Work out the finished part from the listing and answer in its coordinate system (mm). Coordinates: 2 decimals unless noted, no trailing zeros. Write each loop counter-clockwise with the first axis right and the second up, starting at its lowest first coordinate (ties: lowest second). Pieces come first, ordered by that corner, then holes. Notation, with made-up numbers: (1.5, -39) - (42.5, -39) arc R18 cw to (42.5, -26) - close; hole circle Ø6 at (78.5, 80.25). An arc over 180 degrees is marked (long way). Use a Markdown table: item, result. Add a question column.
(1) The part is cut by section C-C, the plane z = 1.55. Give the vertices of the cut face in (x, y), then the cut area to 3 significant figures.
(2) The part is cut by section A-A, the plane y = 0. Give the vertices of the cut face in (x, z), then the cut area to 3 significant figures.
(3) Find the intervals of material crossed by line 1 (Y direction, x = 0, z = 0.8); line 2 (Y direction, x = -30, z = 1.05); line 3 (X direction, y = -8, z = 2.4), in increasing order. Write a range as from..to.
(4) Given pin 1 Ø1.5 at (y, z) = (-8.5, 2) entering from -X; pin 2 Ø0.8 at (y, z) = (13.5, 1.5) entering from -X; pin 3 Ø1.2 at (y, z) = (11, 1) entering from +X, each flat-ended and moving along its own axis, determine where each tip first touches the part or whether it passes through.
(5) The part is cut by section D-D, the plane x = 9.5. Give the vertices of the cut face in (y, z).
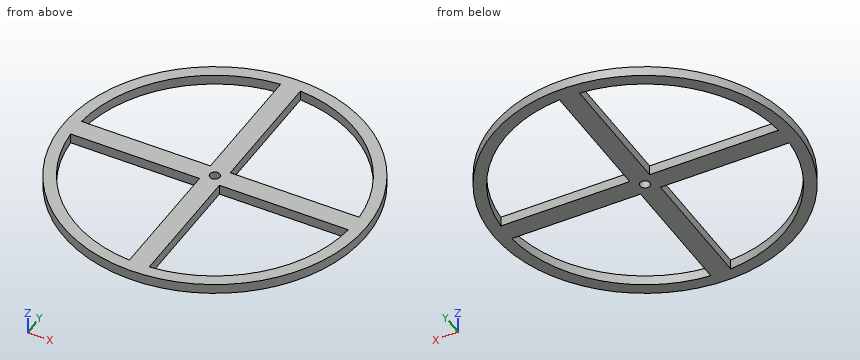
from build123d import *

# Parameters (mm, degrees)
F0_R     = 38
F0_R_2   = 1.25
F1_DEPTH = 2.5


with BuildPart() as f1:
    # F0 (on Top) → F1 (new body)
    with BuildSketch(Plane.XY):
        Circle(F0_R)
        with BuildLine():
            Line((-34.9106, -2.5), (-2.5, -2.5))
            Line((-2.5, -2.5), (-2.5, -34.9106))
            ThreePointArc((-2.5, -34.9106), (-24.748737, -24.748737), (-34.9106, -2.5))
        make_face(mode=Mode.SUBTRACT)
        with BuildLine():
            Line((2.5, -34.9106), (2.5, -2.5))
            Line((2.5, -2.5), (34.9106, -2.5))
            ThreePointArc((34.9106, -2.5), (24.748737, -24.748737), (2.5, -34.9106))
        make_face(mode=Mode.SUBTRACT)
        with BuildLine():
            ThreePointArc((-34.9106, 2.5), (-24.748737, 24.748737), (-2.5, 34.9106))
            Line((-2.5, 34.9106), (-2.5, 2.5))
            Line((-2.5, 2.5), (-34.9106, 2.5))
        make_face(mode=Mode.SUBTRACT)
        Circle(F0_R_2, mode=Mode.SUBTRACT)
        with BuildLine():
            Line((2.5, 2.5), (2.5, 34.9106))
            ThreePointArc((2.5, 34.9106), (24.748737, 24.748737), (34.9106, 2.5))
            Line((34.9106, 2.5), (2.5, 2.5))
        make_face(mode=Mode.SUBTRACT)
    extrude(amount=F1_DEPTH)


solid = f1.part
Model answer:
| question | item | result |
|---|---|---|
| 1 | outline | circle Ø76 at (0, 0); hole (-34.91, -2.5) arc R35 ccw to (-2.5, -34.91) - (-2.5, -2.5) - close; hole (-34.91, 2.5) - (-2.5, 2.5) - (-2.5, 34.91) arc R35 ccw to start; hole circle Ø2.5 at (0, 0); hole (2.5, -34.91) arc R35 ccw to (34.91, -2.5) - (2.5, -2.5) - close; hole (2.5, 2.5) - (34.91, 2.5) arc R35 ccw to (2.5, 34.91) - close |
| 1 | area | 1,360 mm^2 |
| 2 | outline | (-38, 0) - (-1.25, 0) - (-1.25, 2.5) - (-38, 2.5) - close; (1.25, 0) - (38, 0) - (38, 2.5) - (1.25, 2.5) - close |
| 2 | area | 184 mm^2 |
| 3 | line 1 | -38..-1.25, 1.25..38 |
| 3 | line 2 | -23.32..-18.03, -2.5..2.5, 18.03..23.32 |
| 3 | line 3 | -37.15..-34.07, -2.5..2.5, 34.07..37.15 |
| 4 | pin 1 | x = -37.2 |
| 4 | pin 2 | x = -35.67 |
| 4 | pin 3 | x = 36.55 |
| 5 | outline | (-36.79, 0) - (-33.69, 0) - (-33.69, 2.5) - (-36.79, 2.5) - close; (-2.5, 0) - (2.5, 0) - (2.5, 2.5) - (-2.5, 2.5) - close; (33.69, 0) - (36.79, 0) - (36.79, 2.5) - (33.69, 2.5) - close |
